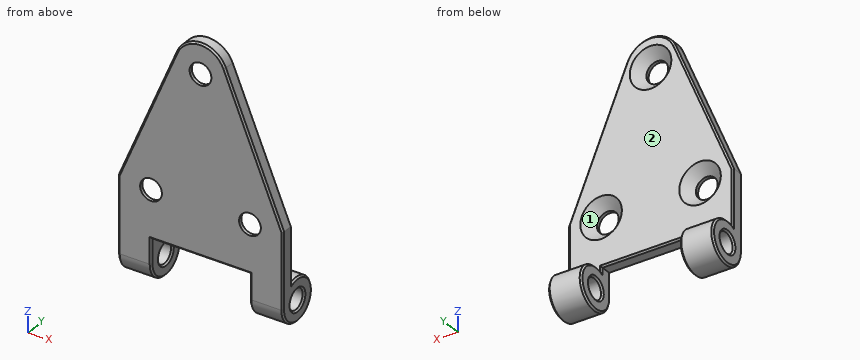
```python
from build123d import *

# Parameters (mm, degrees)
SKETCH1_R                                       = 3.05
BOSS_EXTRUDE1_DEPTH                             = 25
SKETCH2_W                                       = 29.8
SKETCH2_H                                       = 20
CUT_EXTRUDE1_DEPTH                              = 76.45859792
CSK_FOR_M6_FLAT_HEAD_MACHINE_SCREW1_D           = 6.6
CSK_FOR_M6_FLAT_HEAD_MACHINE_SCREW1_DEPTH       = 38.017159957
CSK_FOR_M6_FLAT_HEAD_MACHINE_SCREW1_CSINK_D     = 12.6
CSK_FOR_M6_FLAT_HEAD_MACHINE_SCREW1_CSINK_ANGLE = 90
CSK_FOR_M6_FLAT_HEAD_MACHINE_SCREW1_TIP         = 1.982840043
CHAMFER1_SIZE                                   = 0.5
CHAMFER2_SIZE                                   = 0.5


with BuildPart() as part:
    # Sketch1 → Boss-Extrude1 (new, symmetric)
    with BuildSketch(Plane(origin=(0, 0, 0), x_dir=(0, 0, -1), z_dir=(1, 0, 0))):
        with BuildLine():
            Line((0, 0), (-70, 0))
            Line((-70, 0), (-70, 4))
            Line((-70, 4), (-6, 4))
            ThreePointArc((-6, 4), (3.605551275, 11.908326913), (0, 0))
        make_face()
        with Locations((0, 6.5)):
            Circle(SKETCH1_R, mode=Mode.SUBTRACT)
    extrude(amount=BOSS_EXTRUDE1_DEPTH, both=True)

    # Sketch2 → Cut-Extrude1 (cut, through all)
    with BuildSketch(Plane(origin=(0, 0, 0), x_dir=(1, 0, 0), z_dir=(0, 1, 0))):
        with Locations((0, 2.5)):
            Rectangle(SKETCH2_W, SKETCH2_H)
        with BuildLine():
            Line((-25, -23), (-7.379416922, -65.089369822))
            ThreePointArc((-7.379416922, -65.089369822), (0, -70), (7.379416922, -65.089369822))
            Line((7.379416922, -65.089369822), (25, -23))
            Line((25, -23), (25, -80))
            Line((25, -80), (-25, -80))
            Line((-25, -80), (-25, -23))
        make_face()
    extrude(amount=CUT_EXTRUDE1_DEPTH, mode=Mode.SUBTRACT)

    # CSK for M6 Flat Head Machine Screw1
    with Locations(Plane(origin=(0, 4, 0), x_dir=(1, 0, 0), z_dir=(0, 1, 0))):
        with Locations((15, -22), (-15, -22), (0, -61)):
            CounterSinkHole(CSK_FOR_M6_FLAT_HEAD_MACHINE_SCREW1_D / 2, CSK_FOR_M6_FLAT_HEAD_MACHINE_SCREW1_CSINK_D / 2, depth=CSK_FOR_M6_FLAT_HEAD_MACHINE_SCREW1_DEPTH, counter_sink_angle=CSK_FOR_M6_FLAT_HEAD_MACHINE_SCREW1_CSINK_ANGLE)
            with Locations((0, 0, -(CSK_FOR_M6_FLAT_HEAD_MACHINE_SCREW1_DEPTH + CSK_FOR_M6_FLAT_HEAD_MACHINE_SCREW1_TIP / 2))):  # 118° drill point
                Cone(0, CSK_FOR_M6_FLAT_HEAD_MACHINE_SCREW1_D / 2, CSK_FOR_M6_FLAT_HEAD_MACHINE_SCREW1_TIP, mode=Mode.SUBTRACT)

    # Chamfer1
    chamfer1_edges = [part.edges().sort_by_distance(p)[0] for p in [
        (-25, 6.5, 3.05),
        (25, 6.5, 3.05),
        (-14.9, 6.5, 3.05),
        (14.9, 6.5, 3.05),
    ]]
    chamfer(chamfer1_edges, length=CHAMFER1_SIZE)

    # Chamfer2
    chamfer2_edges = [part.edges().sort_by_distance(p)[0] for p in [
        (-25, 0, 11.5),
        (25, 0, 11.5),
        (0, 0, 70),
        (0, 0, 7.5),
        (-14.9, 0, 3.75),
        (-14.9, 11.908326913, -3.605551275),
        (14.9, 0, 3.75),
        (14.9, 11.908326913, -3.605551275),
        (-14.9, 4, 6.75),
        (0, 4, 7.5),
        (14.9, 4, 6.75),
        (16.189708461, 0, 44.044684911),
        (-16.189708461, 0, 44.044684911),
        (16.189708461, 4, 44.044684911),
        (25, 11.908326913, -3.605551275),
        (0, 4, 70),
        (-16.189708461, 4, 44.044684911),
        (-25, 4, 14.5),
        (-25, 11.908326913, -3.605551275),
        (25, 4, 14.5),
    ]]
    chamfer(chamfer2_edges, length=CHAMFER2_SIZE)


solid = part.part
```
Design review of the part built by this model. Coordinates are the model's own, in mm. Face numbers are marked on the shaded views. Coordinates: 2 decimals unless noted, no trailing zeros. Write each loop counter-clockwise with the first axis right and the second up, starting at its lowest first coordinate (ties: lowest second). Pieces come first, ordered by that corner, then holes. Notation, with made-up numbers: M -20,5 L 9,5 A29 ccw 9,26 Z; hole C 88.5,16.25 d6. An arc over 180 degrees is marked long. Answer as a JSON object with one key per item and string values.
Item 1: Draft analysis for pull direction X (two halves, no side actions). For the marked faces 1 and 2, state which applies: pulls with the +X half, pulls with the -X half, needs draft (parallel to the pull), parting line crosses it, or undercut.
Outcome:
{"face 1": "undercut", "face 2": "needs draft"}
Item 2: Insertion check: pin 1 Ø3.5 at (y, z) = (6.5, 0) entering from +X; pin 2 Ø3.5 at (x, y) = (-3, 1.5) entering from -Z; pin 3 Ø4 at (x, y) = (18.5, 10) entering from +Z. Each pin has a flat end and moves straight along its axis. Give the tip position at first contact, or say it passes through.
Outcome:
{"pin 1": "through", "pin 2": "z = 7.5", "pin 3": "z = 6.32"}
Item 3: Add section C-C, the plane z = 22. Give the boundary of the cut face in (x, y), and give its area (3 significant figures).
Outcome:
{"outline": "M -25,0.5 L -24.5,0 L -18.3,0 L -18.3,1 L -21.3,4 L -24.5,4 L -25,3.5 Z; M -11.7,0 L 11.7,0 L 11.7,1 L 8.7,4 L -8.7,4 L -11.7,1 Z; M 18.3,0 L 24.5,0 L 25,0.5 L 25,3.5 L 24.5,4 L 21.3,4 L 18.3,1 Z", "area": "129 mm²"}
Item 4: Wall thickness on probe 1 along Z at (x, y) = (0, 0.6); probe 2 along Y at (x, z) = (-18, 0); probe 3 along Z at (x, y) = (19.5, 6.5): over which ranges is each line inside the solid? List them lowest first.
Outcome:
{"probe 1": "7.5 to 57.7, 64.3 to 70", "probe 2": "0 to 3.45, 9.55 to 13", "probe 3": "-6.5 to -3.05, 3.05 to 6.5"}
Item 5: Add section A-A, the plane y = 6.5. State how many separate pieces and enclosed holes the cut face has, and give its area (3 significant figures).
Outcome:
{"separate pieces": "4", "enclosed holes": "0", "area": "137 mm²"}
Item 6: Add section D-D, the plane z = 53.5. Give the boundary of the cut face in (x, y).
Outcome:
{"outline": "M -12.23,0.5 L -11.69,0 L 11.69,0 L 12.23,0.5 L 12.23,3.5 L 11.69,4 L -11.69,4 L -12.23,3.5 Z"}
Item 7: Add section B-B, the plane x = 0. Give the boundary of the cut face in (y, z).
Outcome:
{"outline": "M 0,8 L 0.5,7.5 L 3.5,7.5 L 4,8 L 4,54.7 L 1,57.7 L 0,57.7 Z; M 0,64.3 L 1,64.3 L 4,67.3 L 4,69.5 L 3.5,70 L 0.5,70 L 0,69.5 Z"}
